Design review of the part built by this model. Coordinates are the model's own, in mm. Face numbers are marked on the shaded views. A direction names the side the tool comes from. Round coordinates to 2 decimals unless told otherwise and drop trailing zeros. Loops run counter-clockwise (first coordinate to the right, second up) from the corner with the lowest first, then second, coordinate; pieces in that order, holes last. Notation, with made-up numbers: (12, 49.25) -> (48, 49.25) arc R19 cw to (48, 53.25) -> close; hole circle Ø1 at (78, -2). An arc over 180 degrees is marked (long way). Answer as CSV lines item,"result". Start each with the question number.
(1) Take a section at A-A, the plane y = 11. Write out the cut boundary in (x, z), and give its area (3 significant figures).
(2) Machinability: for the marked faces 1, 2 and 3, which of the approach directions +Z, -Z, +X, -X, +Y, -Y give a long, thin tool a straight path to every point of the face, cutting with its end or side? Answer none if there is none.
(3) For P1, Ø4, axis at x = 64, z = -43, coming from the -Y side; P2, Ø1.5, axis at x = 34.5, y = 10.5, coming from the -Z side; P3, Ø7.5, axis at x = 8.5, y = 42, coming from the +Z side, all flat-tipped, find the tip position at first contact; note any pin that passes through.
(4) Take a section at B-B, the plane z = -32.5. Write out the cut boundary in (x, y).
(5) To check wall thickness, follow line 1 (X direction, y = 36, z = -33.5); line 2 (X direction, y = 14, z = -16.5); line 3 (X direction, y = 12, z = -74.5). State the ranges of each line that lie inside material, in increasing order. Write a range as from..to.
(6) Take a section at C-C, the plane x = 24. Write out the cut boundary in (y, z).
(7) Take a section at D-D, the plane x = -61.5. Write out the cut boundary in (y, z), and give its area (3 significant figures).
(8) Draft analysis for pull direction X (two halves, no side actions). For the marked faces 4, 5 and 6, state which applies: +X half, -X half, draft (parallel to the pull), parting line (faces both ways), or undercut.
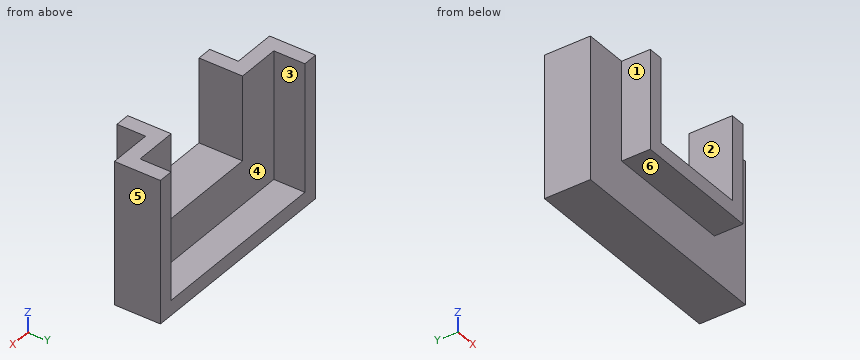
from build123d import *


with BuildPart() as part:
    # Sweep1: sweep along a path in Sketch2
    with BuildLine(Plane(origin=(0, 0, 0), x_dir=(1, 0, 0), z_dir=(0, 1, 0))) as sweep1_path:
        Line((-40, 0), (-40, 68))
        Line((-40, 68), (40, 68))
        Line((40, 68), (40, 0))
    # Sketch3 → Sweep1 (sweep)
    with BuildSketch(Plane.XY):
        Polygon((40, 0), (40, 35), (75, 35), (75, 60), (87, 60), (87, 23), (52, 23), (52, 0), align=None)
    sweep(path=sweep1_path.line, transition=Transition.RIGHT)


solid = part.part
The answers:
1,outline,"(-52, -80) -> (52, -80) -> (52, 0) -> (40, 0) -> (40, -68) -> (-40, -68) -> (-40, 0) -> (-52, 0) -> close"
1,area,"2,880 mm²"
2,face 1,"+Z, -Z, -X, -Y"
2,face 2,"+Z, +Y, -Y"
2,face 3,"+Z, +Y"
3,P1,"y = 23"
3,P2,"z = -80"
3,P3,"z = -103"
4,outline,"(-87, 23) -> (-52, 23) -> (-52, 0) -> (-40, 0) -> (-40, 35) -> (-75, 35) -> (-75, 60) -> (-87, 60) -> close; (40, 0) -> (52, 0) -> (52, 23) -> (87, 23) -> (87, 60) -> (75, 60) -> (75, 35) -> (40, 35) -> close"
5,line 1,"-87..-75, 75..87"
5,line 2,"-52..-40, 40..52"
5,line 3,"-52..52"
6,outline,"(0, -80) -> (23, -80) -> (23, -115) -> (60, -115) -> (60, -103) -> (35, -103) -> (35, -68) -> (0, -68) -> close"
7,outline,"(23, -115) -> (60, -115) -> (60, -103) -> (35, -103) -> (35, 0) -> (23, 0) -> close"
7,area,"1,680 mm²"
8,face 4,"undercut"
8,face 5,"+X half"
8,face 6,"draft"
